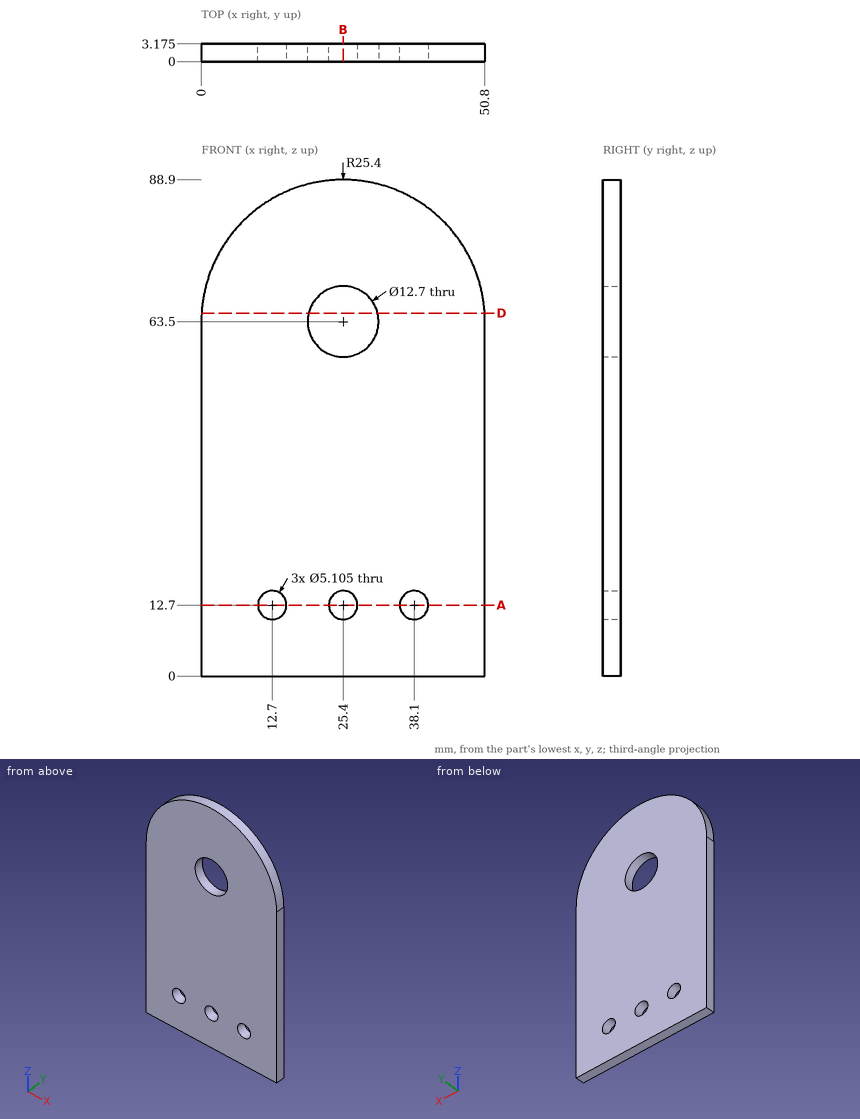
Job drawing, mm, ordinate dimensions from the low corner. One solid piece. Give positions to 0.01 mm unless a question says otherwise; leave off trailing zeros. Loops run counter-clockwise (first coordinate to the right, second up) from the corner with the lowest first, then second, coordinate; pieces in that order, holes last.
Item 1: Slice it at B-B, the plane x = 25.4. Give the number of separate pieces and of enclosed holes in the cut face, and give its area (3 significant figures).
Answers follow:
separate pieces: 3
enclosed holes: 0
area: 226 mm2
Item 2: Drill centre lines: line 1 (Z direction, x = 25.4, y = 2.5); line 2 (Z direction, x = 25, y = 2.7); line 3 (Z direction, x = 22, y = 1.5). Where is each one in solid material? Low to high.
Answers follow:
line 1: z = 0 to 10.15, 15.25 to 57.15, 69.85 to 88.9
line 2: z = 0 to 10.18, 15.22 to 57.16, 69.84 to 88.9
line 3: z = 0 to 58.14, 68.86 to 88.67
Item 3: Flat gauge pins, fed straight in: pin 1 (1.5 mm diameter, centred on x = 5.5, y = 2.5, fed in from +Z) (1 decimal); pin 2 (20.5 mm diameter, centred on x = 25.4, z = 63.5, fed in from -Y); pin 3 (3 mm diameter, centred on x = 38.1, z = 12.7, fed in from -Y). Where does each tip first touch, or does it go through?
Answers follow:
pin 1: stops at z = 80.2
pin 2: stops at y = 0
pin 3: passes through
Item 4: Slice it at A-A, the plane z = 12.7. List the corners of the cut face in (x, y) (1 decimal).
Answers follow:
outline: (0, 0) - (10.1, 0) - (10.1, 3.2) - (0, 3.2) - close; (15.3, 0) - (22.8, 0) - (22.8, 3.2) - (15.3, 3.2) - close; (28, 0) - (35.5, 0) - (35.5, 3.2) - (28, 3.2) - close; (40.7, 0) - (50.8, 0) - (50.8, 3.2) - (40.7, 3.2) - close
Item 5: Slice it at D-D, the plane z = 65. List the corners of the cut face in (x, y) (1 decimal), and give its area (3 significant figures).
Answers follow:
outline: (0, 0) - (19.2, 0) - (19.2, 3.2) - (0, 3.2) - close; (31.6, 0) - (50.8, 0) - (50.8, 3.2) - (31.6, 3.2) - close
area: 122 mm2
